Read the model definition and answer for the solid it produces. Units are mm, in the model's axes. Face numbers are marked on the shaded views. A direction names the side the tool comes from. Coordinates: 2 decimals unless noted, no trailing zeros. Loops run counter-clockwise (first coordinate to the right, second up) from the corner with the lowest first, then second, coordinate; pieces in that order, holes last. Notation, with made-up numbers: (-9.75, 42) - (12.25, 42) arc R13 ccw to (12.25, 47) - close; hole circle Ø6 at (-7.75, 20.25). An arc over 180 degrees is marked (long way). Use one line per item in the form item = value. Start each with the question number.
1) A cutting plane is placed at A-A (x = 0). Give the vertices of the cut face in (y, z), and give its area (3 significant figures).
2) A cutting plane is placed at B-B (z = 0). Give the vertices of the cut face in (x, y), and give its area (3 significant figures).
3) A cutting plane is placed at C-C (y = 3.5). Give the vertices of the cut face in (x, z), and give its area (3 significant figures).
4) Which of the six approach directions +Z, -Z, +X, -X, +Y, -Y give full straight-line access (tool end or side, diameter ignored) to the marked faces 4, 5 and 6?
5) Consider line 1 (Z direction, x = 0, y = 19.75); line 2 (Y direction, x = -2, z = 1); line 3 (Z direction, x = 0, y = 8.25). Determine where each line is inside the solid, lowest interval first.
6) A cutting plane is placed at D-D (z = -2.5). Give the vertices of the cut face in (x, y).
7) The mould has two halves that part along Y. Classify the marked faces 1, 2 and 3: released by +Y, released by -Y, zero draft, split by the parting line, or undercut.
8) Each of these flat-tipped pins is pushed along its axis until it touches: P1, Ø1.9, axis at x = 0, z = 0.5, coming from the +Y side; P2, Ø2, axis at x = 2, y = 12, coming from the -Z side. Where does it stop, or does it pass through?
Autodesk Inventor part; units mm, degrees
ref_plane "YZ Plane" through (0, 0, 0) normal (1, 0, 0) x (0, 1, 0)
ref_plane "XZ Plane" through (0, 0, 0) normal (0, 1, 0) x (-1, 0, 0)
ref_plane "XY Plane" through (0, 0, 0) normal (0, 0, 1) x (1, 0, 0)
sketch "Sketch1" plane through (0, 0, 0) normal (0, 0, 1) x (1, 0, 0)
  line L0 (0, 0) -> (2.8, 0)
  line L1 (2.8, 0) -> (2.8, 5)
  line L2 (2.8, 5) -> (1.4, 5)
  line L3 (1.4, 5) -> (1.4, 7.1)
  line L4 (1.4, 7.1) -> (3.3, 7.1)
  line L5 (3.3, 7.1) -> (3.3, 21.9)
  line L6 (3.3, 21.9) -> (0, 21.9)
  line L7 (0, 21.9) -> (0, 0)
  dimension "d0" = 2.8
  dimension "d1" = 5
  dimension "d2" = 1.4
  dimension "d3" = 2.1
  dimension "d4" = 3.3
  dimension "d5" = 14.8
revolve "Revolution1" add sketch "Sketch1" angle 360 about axis through (0, 21.9, 0) along (0, -1, 0)
thread "Thread1"
sketch "Sketch2" plane through (0, 0, 0) normal (0, -1, 0) x (1, 0, 0)
  circle A0 centre (0, 0) radius 3.3
  circle A1 centre (0, 0) radius 1
  dimension "d11" = 2
extrude "Extrusion1" cut sketch "Sketch2" against normal up to surface (21.9 mm away) contours A1
sketch "Sketch3" plane through (0, 21.9, 0) normal (0, 1, 0) x (1, 0, 0)
  circle A0 centre (0, 0) radius 1
  circle A1 centre (0, 0) radius 3.3
  circle A2 centre (0, 0) radius 1.9
  dimension "d14" = 3.8
extrude "Extrusion2" cut sketch "Sketch3" against normal blind 10.5 contours A2
properties part number "ChimeraHeatBreak" material "Stainless Steel"
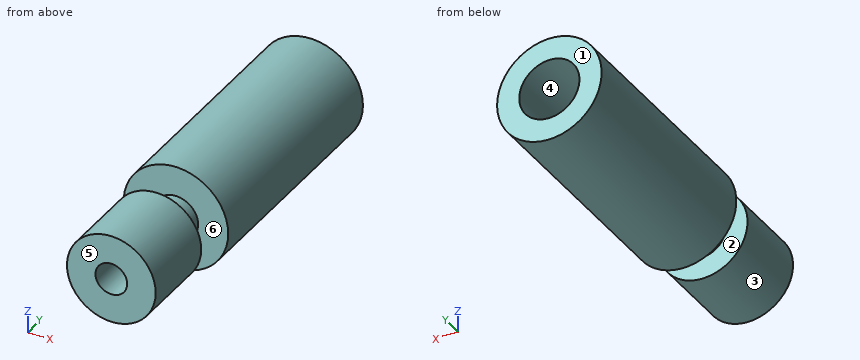
Found:
q1.outline = (0, -2.8) - (5, -2.8) - (5, -1.4) - (7.1, -1.4) - (7.1, -3.3) - (21.9, -3.3) - (21.9, -1.9) - (11.4, -1.9) - (11.4, -1) - (0, -1) - close; (0, 1) - (11.4, 1) - (11.4, 1.9) - (21.9, 1.9) - (21.9, 3.3) - (7.1, 3.3) - (7.1, 1.4) - (5, 1.4) - (5, 2.8) - (0, 2.8) - close
q1.area = 68.9 mm^2
q2.outline = (-3.3, 7.1) - (-1.4, 7.1) - (-1.4, 5) - (-2.8, 5) - (-2.8, 0) - (-1, 0) - (-1, 11.4) - (-1.9, 11.4) - (-1.9, 21.9) - (-3.3, 21.9) - close; (1, 0) - (2.8, 0) - (2.8, 5) - (1.4, 5) - (1.4, 7.1) - (3.3, 7.1) - (3.3, 21.9) - (1.9, 21.9) - (1.9, 11.4) - (1, 11.4) - close
q2.area = 68.9 mm^2
q3.outline = circle Ø5.6 at (0, 0); hole circle Ø2 at (0, 0)
q3.area = 21.5 mm^2
q4.face_4 = +Y
q4.face_5 = +Z, -Z, +X, -X, -Y
q4.face_6 = none
q5.line_1 = -3.3 to -1.9, 1.9 to 3.3
q5.line_2 = 0 to 5, 7.1 to 21.9
q5.line_3 = -3.3 to -1, 1 to 3.3
q6.outline = (-2.15, 7.1) - (2.15, 7.1) - (2.15, 21.9) - (-2.15, 21.9) - close; (-1.26, 0) - (1.26, 0) - (1.26, 5) - (-1.26, 5) - close
q7.face_1 = released by +Y
q7.face_2 = undercut
q7.face_3 = zero draft
q8.P1 = 11.4
q8.P2 = -3.14
